Source: three-view drawing plus pictorial views. Frame: mm from the lowest corner of the part. A direction names the side the tool comes from. Give positions to 0.01 mm unless a question says otherwise; leave off trailing zeros. Order: outer loops, then holes, each group sorted by start corner. A loop starts at its lowest first (then second) coordinate and runs counter-clockwise, first axis right, second up. Notation, with made-up numbers: (5, 40) - (28, 40) arc R11 cw to (28, 44) - close; hole circle Ø2 at (88, 45.5). An arc over 180 degrees is marked (long way). Use one line per item in the form item = value.
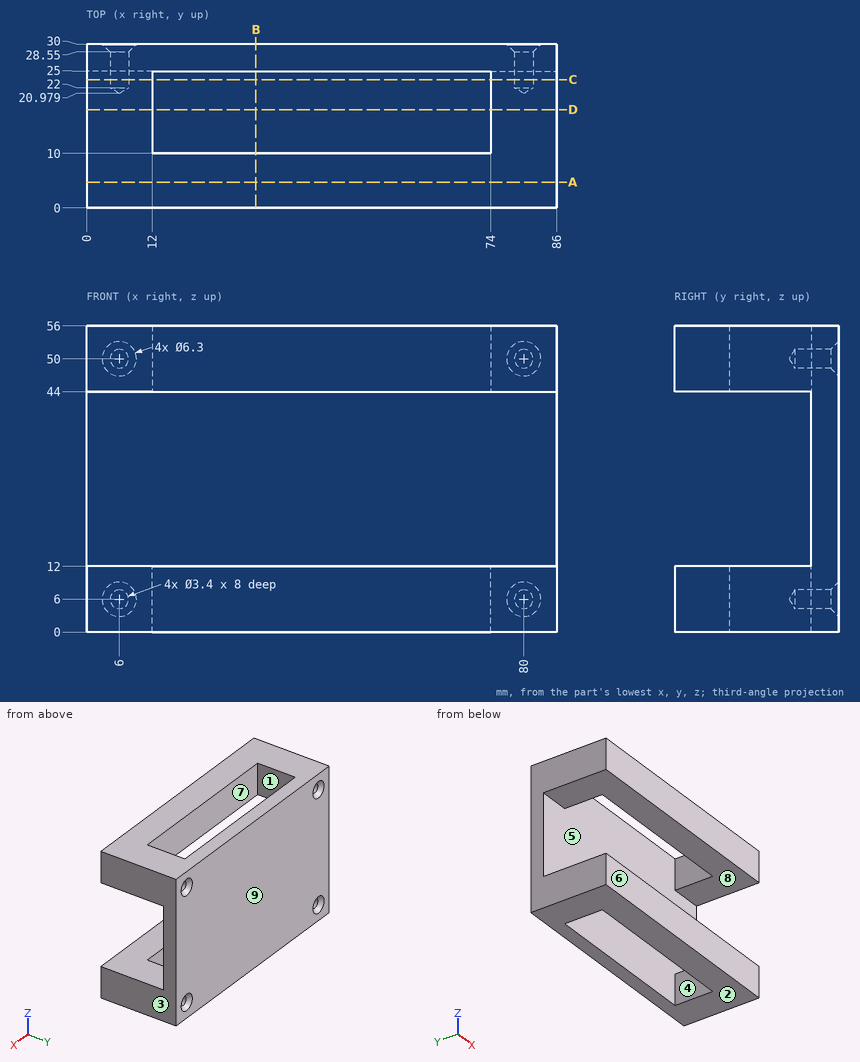
(1) Cut plane B-B on x = 31. Output: boundary loops of the cut face in (y, z), plus the area to 3 significant figures.
Computed values:
outline = (0, 0) - (10, 0) - (10, 12) - (0, 12) - close; (0, 44) - (10, 44) - (10, 56) - (0, 56) - close; (25, 0) - (30, 0) - (30, 56) - (25, 56) - close
area = 520 mm²
(2) Cut plane A-A on y = 4.75. Output: boundary loops of the cut face in (x, z), plus the area to 3 significant figures.
Computed values:
outline = (0, 0) - (86, 0) - (86, 12) - (0, 12) - close; (0, 44) - (86, 44) - (86, 56) - (0, 56) - close
area = 2,060 mm²
(3) Ray query, line 1 along X through (y, z) = (25.75, 50); line 2 along X through (y, z) = (24.25, 50); line 3 along Y through (x, z) = (71.5, 49). Return the intervals inside material, ascending.
Computed values:
line_1 = 0 to 4.3, 7.7 to 78.3, 81.7 to 86
line_2 = 0 to 4.3, 7.7 to 12, 74 to 78.3, 81.7 to 86
line_3 = 0 to 10, 25 to 30
(4) Cut plane C-C on y = 23.5. Output: boundary loops of the cut face in (x, z).
Computed values:
outline = (0, 0) - (12, 0) - (12, 12) - (0, 12) - close; (0, 44) - (12, 44) - (12, 56) - (0, 56) - close; (74, 0) - (86, 0) - (86, 12) - (74, 12) - close; (74, 44) - (86, 44) - (86, 56) - (74, 56) - close; hole circle Ø3.4 at (6, 6); hole circle Ø3.4 at (6, 50); hole circle Ø3.4 at (80, 6); hole circle Ø3.4 at (80, 50)
(5) Pull-direction query (X, two-part tool) for the marked faces 1, 2, 3 and 4; classes: released by +X, released by -X, zero draft, split by the parting line, or undercut.
Computed values:
face_1 = undercut
face_2 = zero draft
face_3 = released by +X
face_4 = undercut
(6) Cut plane D-D on y = 18. Output: boundary loops of the cut face in (x, z).
Computed values:
outline = (0, 0) - (12, 0) - (12, 12) - (0, 12) - close; (0, 44) - (12, 44) - (12, 56) - (0, 56) - close; (74, 0) - (86, 0) - (86, 12) - (74, 12) - close; (74, 44) - (86, 44) - (86, 56) - (74, 56) - close
(7) Contact query for flat-ended pins moving along their axis: pin 1 Ø2 at (x, z) = (6, 50) entering from +Y; pin 2 Ø3 at (x, z) = (6, 6) entering from +Y; pin 3 Ø2.5 at (x, z) = (80, 6) entering from +Y. Output: stop coordinate, or through.
Computed values:
pin_1 = 21.58
pin_2 = 21.88
pin_3 = 21.73
(8) Reachability of the marked faces 5, 6, 7, 8 and 9 from +Z, -Z, +X, -X, +Y, -Y: full face, straight path, thin tool, end or side. Return the list, or none.
Computed values:
face_5 = none
face_6 = +Z, -Z, +X, -X, -Y
face_7 = +Z, -Z
face_8 = +X, -X, -Y
face_9 = +Z, -Z, +X, -X, +Y
